from build123d import *

# Parameters (mm, degrees)
RESSALTO_EXTRUS_O1_DEPTH         = 35
FURO_DE_DI_METRO_11_0_11_1_D     = 11
FUROS_GUIA_COM_10_0MM1_D         = 10
FURO_DE_DI_METRO_11_0_11_2_D     = 11
FURO_DE_DI_METRO_11_0_11_2_DEPTH = 10
FURO_DE_DI_METRO_11_0_11_2_TIP   = 3.304733405


with BuildPart() as part:
    # Esboço1 → Ressalto-extrusão1 (new body)
    with BuildSketch(Plane.XY):
        with BuildLine():
            Line((-199.997669575, -240.109131808), (-34.994179097, -240.27276126))
            ThreePointArc((-34.994179097, -240.27276126), (-0.031980607, -274.807449281), (34.998643265, -240.34217123))
            Line((34.998643265, -240.34217123), (200.002133743, -240.505800682))
            Line((200.002133743, -240.505800682), (199.972879413, -270.005786177))
            Line((199.972879413, -270.005786177), (57.635762375, -269.864634348))
            ThreePointArc((57.635762375, -269.864634348), (-0.061730772, -304.80743453), (-57.689806866, -269.750269132))
            Line((-57.689806866, -269.750269132), (-200.026923904, -269.609117302))
            Line((-200.026923904, -269.609117302), (-199.997669575, -240.109131808))
        make_face()
    extrude(amount=-RESSALTO_EXTRUS_O1_DEPTH)

    # Furo de diâmetro Ø11.0 (11)1 (through all)
    with Locations(Plane(origin=(-0.238306111, -240.30722771, 0), x_dir=(0.9999995082930158, -0.000991672187112085, 0), z_dir=(0.000991672187112085, 0.9999995082930158, 0))):
        with Locations((-179.759461687, 17.5), (-79.759461687, 17.5), (80.240538313, 17.5), (180.240538313, 17.5)):
            Hole(FURO_DE_DI_METRO_11_0_11_1_D / 2)

    # Furos-guia com Ø10.0mm1 (through all)
    with Locations(Plane(origin=(-0.267560441, -269.807213205, 0), x_dir=(-0.9999995082930158, 0.0009916721871120312, 0), z_dir=(-0.0009916721871120312, -0.9999995082930158, 0))):
        with Locations((129.759461687, 17.5), (-130.240538313, 17.5), (-221.181262437, -155.418379851)):
            Hole(FUROS_GUIA_COM_10_0MM1_D / 2)

    # Furo de diâmetro Ø11.0 (11)2
    with Locations(Plane(origin=(-0.267560441, -269.807213205, 0), x_dir=(-0.9999995082930158, 0.0009916721871120312, 0), z_dir=(-0.0009916721871120312, -0.9999995082930158, 0))):
        with Locations((129.759461687, 17.5), (-130.240538313, 17.5)):
            Hole(FURO_DE_DI_METRO_11_0_11_2_D / 2, depth=FURO_DE_DI_METRO_11_0_11_2_DEPTH)
            with Locations((0, 0, -(FURO_DE_DI_METRO_11_0_11_2_DEPTH + FURO_DE_DI_METRO_11_0_11_2_TIP / 2))):  # 118° drill point
                Cone(0, FURO_DE_DI_METRO_11_0_11_2_D / 2, FURO_DE_DI_METRO_11_0_11_2_TIP, mode=Mode.SUBTRACT)


solid = part.part
Work out the finished part from the listing and answer in its coordinate system (mm). Round coordinates to 2 decimals unless told otherwise and drop trailing zeros. Loops run counter-clockwise (first coordinate to the right, second up) from the corner with the lowest first, then second, coordinate; pieces in that order, holes last. Notation, with made-up numbers: M -35.75,53.5 L -15.75,53.5 A17 cw -15.75,85.5 Z; hole C 4,48.5 d2. An arc over 180 degrees is marked long. One line per question, with ' | ' between items. Start each with the question number.
(1) A cutting plane is placed at C-C on x = -14. Write down the section's boundary in (y, z).
(2) Flat-ended cylindrical pins translate along their axes: pin 1 Ø6 at (x, z) = (-53.5, -6.5) entering from -Y; pin 2 Ø4 at (x, z) = (-36.5, -4) entering from +Y; pin 3 Ø6 at (x, z) = (-91, -22) entering from +Y; pin 4 Ø10 at (x, y) = (44.5, -253) entering from +Z. Find the tip coordinate at first contact, or state that the pin passes through.
(3) A cutting plane is placed at B-B on y = -283.5. Write down the section's boundary in (x, z), plus the area to 3 significant figures.
(4) For a pull along X with two mould halves and no side action, classify faces 1 (the face through (3, -279, 0)), 2 (the face through (0.9, -304.8, -17.3)), 3 (the face through (-185.09, -255.08, -15.39)) as released by +X, released by -X, zero draft, split by the parting line, or undercut.
(5) A cutting plane is placed at A-A on z = -28. Write down the section's boundary in (x, y), plus the area to 3 significant figures.
(6) Find the intervals of material crossed by line 1 (Y direction, x = -62, z = -20.5); line 2 (X direction, y = -267, z = -7.5); line 3 (Y direction, x = 114, z = -14), in increasing order.
Geometry check:
1) outline: M -303.28,-35 L -271.88,-35 L -271.88,0 L -303.28,0 Z
2) pin 1: stops at y = -280.73 | pin 2: stops at y = -240.27 | pin 3: stops at y = -240.21 | pin 4: stops at z = 0
3) outline: M -48.12,-35 L 48.13,-35 L 48.13,0 L -48.12,0 Z | area: 3,370 mm²
4) face 1: zero draft | face 2: split by the parting line | face 3: undercut
5) outline: M -200.03,-269.61 L -57.69,-269.75 A65 ccw 57.64,-269.86 L 199.97,-270.01 L 200,-240.51 L 35,-240.34 A35 cw -34.99,-240.27 L -200,-240.11 Z | area: 12,800 mm²
6) line 1: y = -269.75 to -240.25 | line 2: x = -200.02 to -22.03, 22.04 to 199.98 | line 3: y = -269.92 to -240.42
